Source: CAD feature listing. Evaluate the final solid. Frame: model axes, mm. Face numbers are marked on the shaded views. A direction names the side the tool comes from. Round coordinates to 2 decimals unless told otherwise and drop trailing zeros. Write each loop counter-clockwise with the first axis right and the second up, starting at its lowest first coordinate (ties: lowest second). Pieces come first, ordered by that corner, then holes. Notation, with made-up numbers: M 27,38 L 81,38 A32 ccw 81,71 Z; hole C -10,-29.75 d4. An arc over 180 degrees is marked long. Use a Markdown table: item, result.
Autodesk Inventor part; units mm, degrees
ref_plane "YZ Plane" through (0, 0, 0) normal (1, 0, 0) x (0, 1, 0)
ref_plane "XZ Plane" through (0, 0, 0) normal (0, 1, 0) x (-1, 0, 0)
ref_plane "XY Plane" through (0, 0, 0) normal (0, 0, 1) x (1, 0, 0)
sketch "スケッチ1" plane through (0, 0, 0) normal (0, 0, 1) x (1, 0, 0)
  circle A0 centre (0, 0) radius 1.5
  dimension "d0" = 3
extrude "押し出し1" add sketch "スケッチ1" along normal blind 25
thread "ねじ1"
sketch "スケッチ2" plane through (0, 0, 25) normal (0, 0, 1) x (1, 0, 0)
  circle A0 centre (0, 0) radius 3
  dimension "d5" = 6
extrude "押し出し2" add sketch "スケッチ2" against normal blind 1.75
chamfer "面取り1" distance 1.5 angle 45 1 edges at (-3, 0, 23.25)
sketch "スケッチ3" plane through (0, 0, 25) normal (0, 0, 1) x (1, 0, 0)
  line L0 (0, 1.1547) -> (1, 0.5774)
  line L1 (1, 0.5774) -> (1, -0.5774)
  line L2 (1, -0.5774) -> (0, -1.1547)
  line L3 (0, -1.1547) -> (-1, -0.5774)
  line L4 (-1, -0.5774) -> (-1, 0.5774)
  line L5 (-1, 0.5774) -> (0, 1.1547)
  point P0 (0, 0)
  point P1 (0, 0)
  dimension "d11" = 2
extrude "押し出し3" cut sketch "スケッチ3" against normal blind 1.5
properties part number "m3皿ネジ15" material "鉄 灰色"
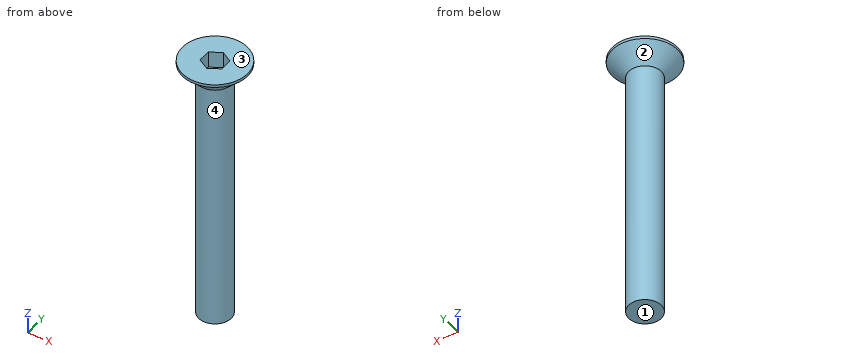
Q1. Mould query, pull axis Y, two halves, no side actions, for the marked faces 1 and 2. Classes: +Y half, -Y half, draft (parallel to the pull), parting line (faces both ways), or undercut.
Results are:
| item | result |
|---|---|
| face 1 | draft |
| face 2 | parting line |
Q2. Line query: L1, parallel to Y at x = 0, z = 9; L2, parallel to Z at x = 0.1, y = 1.75; L3, parallel to Z at x = 0.4, y = -0.15. Output: solid intervals per line, ascending.
Results are:
| item | result |
|---|---|
| L1 | -1.5 to 1.5 |
| L2 | 23.5 to 25 |
| L3 | 0 to 23.5 |
Q3. Section B-B on z = 9. Return loops of the section in (x, y).
Results are:
| item | result |
|---|---|
| outline | C 0,0 d3 |
Q4. First-contact query: pin 1 Ø1 at (y, z) = (-2.5, 2.5) entering from -X; pin 2 Ø1.3 at (y, z) = (0.5, 24) entering from +X; pin 3 Ø2 at (y, z) = (-1.5, 13.5) entering from -X; pin 4 Ø1 at (y, z) = (0.5, 9) entering from -X. Flat tips, straight axial feed; report the tip coordinate or a pass-through.
Results are:
| item | result |
|---|---|
| pin 1 | through |
| pin 2 | x = 2.87 |
| pin 3 | x = -1.41 |
| pin 4 | x = -1.5 |
Q5. Reachability of the marked faces 3 and 4 from +Z, -Z, +X, -X, +Y, -Y: full face, straight path, thin tool, end or side. Return the list, or none.
Results are:
| item | result |
|---|---|
| face 3 | +Z, +X, -X, +Y, -Y |
| face 4 | -Z |
